Could you check a few things on this model? Use its own coordinates, in mm. Face numbers are marked on the shaded views. A direction names the side the tool comes from. Give positions to 0.01 mm unless a question says otherwise; leave off trailing zeros. Write each loop counter-clockwise with the first axis right and the second up, starting at its lowest first coordinate (ties: lowest second). Pieces come first, ordered by that corner, then holes. Notation, with made-up numbers: M -14,-31.75 L 9,-31.75 A32 ccw 9,5.25 Z; hole C -32.5,37.5 d9. An arc over 180 degrees is marked long. Use one line per item in the form item = value.
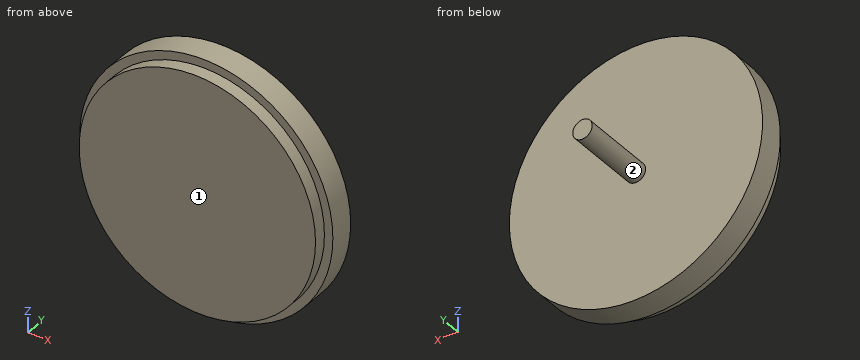
from build123d import *

# Parameters (mm, degrees)
SKETCH_R     = 30
PAD_DEPTH    = 6
SKETCH001_R  = 28
PAD001_DEPTH = 3
SKETCH002_R  = 2.3
PAD002_DEPTH = 18


with BuildPart() as part:
    # Sketch → Pad (new body)
    with BuildSketch(Plane.XZ):
        Circle(SKETCH_R)
    extrude(amount=PAD_DEPTH)

    # Sketch001 (on Face3 of Pad) → Pad001 (join)
    with BuildSketch(Plane.XZ.offset(6)):
        Circle(SKETCH001_R)
    extrude(amount=PAD001_DEPTH)

    # Sketch002 (on Face2 of Pad001) → Pad002 (join)
    with BuildSketch(Plane(origin=(0, 0, 0), x_dir=(1, 0, 0), z_dir=(0, 1, 0))):
        Circle(SKETCH002_R)
    extrude(amount=PAD002_DEPTH)


solid = part.part
1) I want a section at A-A, the plane z = 0. Please give me the cut outline in (x, y), plus the area to 3 significant figures.
Checked values:
outline = M -30,-6 L -28,-6 L -28,-9 L 28,-9 L 28,-6 L 30,-6 L 30,0 L 2.3,0 L 2.3,18 L -2.3,18 L -2.3,0 L -30,0 Z
area = 611 mm2
2) I want a section at C-C, the plane y = 11.5. Please give me the cut outline in (x, z), plus the area to 3 significant figures.
Checked values:
outline = C 0,0 d4.6
area = 16.6 mm2
3) For the marked faces 1 and 2, which set-ups out of +Z, -Z, +X, -X, +Y, -Y let a thin tool reach every point of the face, with its end or its side?
Checked values:
face_1 = +Z, -Z, +X, -X, -Y
face_2 = +Y
4) I want a section at B-B, the plane x = 0. Please give me the cut outline in (y, z).
Checked values:
outline = M -9,-28 L -6,-28 L -6,-30 L 0,-30 L 0,-2.3 L 18,-2.3 L 18,2.3 L 0,2.3 L 0,30 L -6,30 L -6,28 L -9,28 Z
5) I want a section at D-D, the plane z = -13. Please give me the cut outline in (x, y).
Checked values:
outline = M -27.04,-6 L -24.8,-6 L -24.8,-9 L 24.8,-9 L 24.8,-6 L 27.04,-6 L 27.04,0 L -27.04,0 Z
6) If I drill on L1, parallel to Y at x = -6, z = -13.5; L2, parallel to Y at x = -23, z = 19; L3, parallel to Z at x = -0.5, y = 0.5 (3 decimals), over which ranges is the centre line in solid material (lowest first)?
Checked values:
L1 = -9 to 0
L2 = -6 to 0
L3 = -2.245 to 2.245
7) For pin 1 Ø8 at (y, z) = (-5.5, -14) entering from +X; pin 2 Ø2 at (x, z) = (16.5, -6) entering from +Y; pin 3 Ø5 at (x, y) = (1.5, -5) entering from -Z, each with a flat end and sliding along its axis, tell me the tip position at first contact or that it passes through.
Checked values:
pin_1 = 28.28
pin_2 = 0
pin_3 = -30
